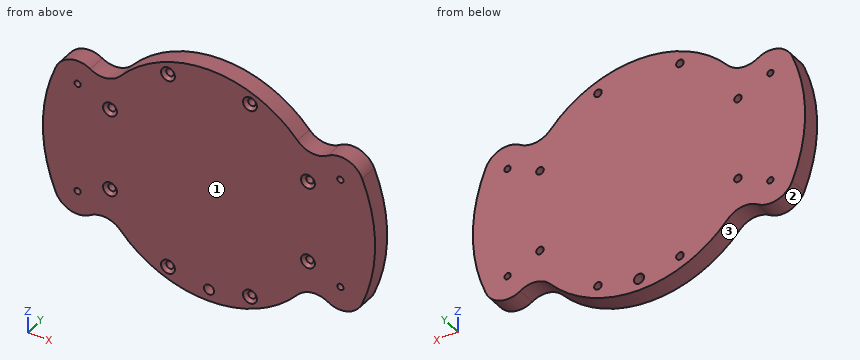
```python
from build123d import *

# Parameters (mm, degrees)
SKETCH1_R                                       = 1
BOSS_EXTRUDE1_DEPTH                             = 6
FILLET1_R                                       = 7.5
SKETCH2_R                                       = 1.6
CUT_EXTRUDE1_DEPTH                              = 66.108380797
CSK_FOR_M2_FLAT_HEAD_MACHINE_SCREW1_D           = 2.4
CSK_FOR_M2_FLAT_HEAD_MACHINE_SCREW1_CSINK_D     = 4.4
CSK_FOR_M2_FLAT_HEAD_MACHINE_SCREW1_CSINK_ANGLE = 90


with BuildPart() as part:
    # Sketch1 → Boss-Extrude1 (new body)
    with BuildSketch(Plane(origin=(0, 0, 0), x_dir=(1, 0, 0), z_dir=(0, 1, 0))):
        with BuildLine():
            Line((31.883633055, 20.164562188), (44.561021943, 28.182280752))
            ThreePointArc((44.561021943, 28.182280752), (52.725, 0), (44.561021943, -28.182280752))
            Line((44.561021943, -28.182280752), (31.883633055, -20.164562188))
            ThreePointArc((31.883633055, -20.164562188), (0, -37.725), (-31.883633055, -20.164562188))
            Line((-31.883633055, -20.164562188), (-44.561021943, -28.182280752))
            ThreePointArc((-44.561021943, -28.182280752), (-52.725, 0), (-44.561021943, 28.182280752))
            Line((-44.561021943, 28.182280752), (-31.883633055, 20.164562188))
            ThreePointArc((-31.883633055, 20.164562188), (0, 37.725), (31.883633055, 20.164562188))
        make_face()
        with Locations(Location((-13.0112367, 31.411904105, 0), (0, 0, 270))):
            Circle(SKETCH1_R, mode=Mode.SUBTRACT)
        with Locations(Location((13.0112367, 31.411904105, 0), (0, 0, 270))):
            Circle(SKETCH1_R, mode=Mode.SUBTRACT)
        with Locations(Location((31.411904105, 13.0112367, 0), (0, 0, 270))):
            Circle(SKETCH1_R, mode=Mode.SUBTRACT)
        with Locations(Location((31.411904105, -13.0112367, 0), (0, 0, 270))):
            Circle(SKETCH1_R, mode=Mode.SUBTRACT)
        with Locations(Location((13.0112367, -31.411904105, 0), (0, 0, 270))):
            Circle(SKETCH1_R, mode=Mode.SUBTRACT)
        with Locations(Location((-13.0112367, -31.411904105, 0), (0, 0, 270))):
            Circle(SKETCH1_R, mode=Mode.SUBTRACT)
        with Locations(Location((-31.411904105, -13.0112367, 0), (0, 0, 270))):
            Circle(SKETCH1_R, mode=Mode.SUBTRACT)
        with Locations(Location((-31.411904105, 13.0112367, 0), (0, 0, 270))):
            Circle(SKETCH1_R, mode=Mode.SUBTRACT)
        with Locations(Location((41.701925915, 17.5, 0), (0, 0, 270))):
            Circle(SKETCH1_R, mode=Mode.SUBTRACT)
        with Locations(Location((41.701925915, -17.5, 0), (0, 0, 270))):
            Circle(SKETCH1_R, mode=Mode.SUBTRACT)
        with Locations(Location((-41.701925915, 17.5, 0), (0, 0, 90))):
            Circle(SKETCH1_R, mode=Mode.SUBTRACT)
        with Locations(Location((-41.701925915, -17.5, 0), (0, 0, 90))):
            Circle(SKETCH1_R, mode=Mode.SUBTRACT)
    extrude(amount=BOSS_EXTRUDE1_DEPTH)

    # Fillet1
    fillet1_edges = [part.edges().sort_by_distance(p)[0] for p in [
        (44.561021943, 3, 28.182280752),
        (31.883633055, 3, 20.164562188),
        (-44.561021943, 3, 28.182280752),
        (-31.883633055, 3, 20.164562188),
        (44.561021943, 3, -28.182280752),
        (31.883633055, 3, -20.164562188),
        (-44.561021943, 3, -28.182280752),
        (-31.883633055, 3, -20.164562188),
    ]]
    fillet(fillet1_edges, radius=FILLET1_R - 0.0001)  # a hair under: the kernel refuses the full size

    # Sketch2 → Cut-Extrude1 (cut, through all)
    with BuildSketch(Plane(origin=(0, 6, 0), x_dir=(1, 0, 0), z_dir=(0, 1, 0))):
        with Locations(Location((0, 34, 0), (0, 0, 270))):
            Circle(SKETCH2_R)
    extrude(amount=-CUT_EXTRUDE1_DEPTH, mode=Mode.SUBTRACT)

    # CSK for M2 Flat Head Machine Screw1 (through all)
    with Locations(Plane(origin=(0, 0, 0), x_dir=(-1, 0, 0), z_dir=(0, -1, 0))):
        with Locations((13.0112367, -31.411904105), (-13.0112367, -31.411904105), (-31.411904105, -13.0112367), (-31.411904105, 13.0112367), (-13.0112367, 31.411904105), (13.0112367, 31.411904105), (31.411904105, 13.0112367), (31.411904105, -13.0112367)):
            CounterSinkHole(CSK_FOR_M2_FLAT_HEAD_MACHINE_SCREW1_D / 2, CSK_FOR_M2_FLAT_HEAD_MACHINE_SCREW1_CSINK_D / 2, counter_sink_angle=CSK_FOR_M2_FLAT_HEAD_MACHINE_SCREW1_CSINK_ANGLE)


solid = part.part
```
The listing builds one solid part. Answer for the finished solid, in the listing's coordinates (mm). Face numbers are marked on the shaded views. Give positions to 0.01 mm unless a question says otherwise; leave off trailing zeros. Write each loop counter-clockwise with the first axis right and the second up, starting at its lowest first coordinate (ties: lowest second). Pieces come first, ordered by that corner, then holes. Notation, with made-up numbers: (3, 68.5) -> (49, 68.5) arc R18 ccw to (49, 91.5) -> close; hole circle Ø7 at (49, 53.25). An arc over 180 degrees is marked (long way). Use one line per item in the form item = value.
1) Each of these flat-tipped pins is pushed along its axis until it touches: P1, Ø4, axis at x = 13.01, z = 31.41, coming from the -Y side; P2, Ø3, axis at y = 2, z = 3, coming from the -X side; P3, Ø1, axis at x = 27.5, y = 4.5, coming from the -Z side. Where does it stop, or does it pass through?
Result:
P1 = 0.2
P2 = -52.7
P3 = -26.35
2) Section A-A on x = 0 is taken. Write down the section's boundary in (y, z) (3 decimals), plus the area to 4 significant figures.
Result:
outline = (0, -37.725) -> (6, -37.725) -> (6, -35.6) -> (0, -35.6) -> close; (0, -32.4) -> (6, -32.4) -> (6, 37.725) -> (0, 37.725) -> close
area = 433.5 mm²
3) For a pull along X with two mould halves and no side action, classify the marked faces 1, 2 and 3 as +X half, -X half, draft (parallel to the pull), parting line (faces both ways), or undercut.
Result:
face_1 = draft
face_2 = undercut
face_3 = parting line
4) Straight lines are drawn through the part: probe 1 along X at (y, z) = (2.8, 17.5); probe 2 along X at (y, z) = (3.85, -13); probe 3 along Z at (x, y) = (-13.5, 2.75). For each, find the intervals that lie inside material, in ascending order.
Result:
probe_1 = -49.74 to -42.7, -40.7 to 40.7, 42.7 to 49.74
probe_2 = -51.1 to -32.61, -30.21 to 30.21, 32.61 to 51.1
probe_3 = -35.23 to -32.51, -30.32 to 30.32, 32.51 to 35.23
5) Section C-C on z = -28 is taken. Write down the section's boundary in (x, y), plus the area to 3 significant figures.
Result:
outline = (-25.28, 0) -> (25.28, 0) -> (25.28, 6) -> (-25.28, 6) -> close
area = 303 mm²
6) Section B-B on y = 4.2 is taken. Count the separate pieces of the cut face and the enclosed holes in it, plus the area to 3 significant figures.
Result:
separate_pieces = 1
enclosed_holes = 13
area = 5,920 mm²
7) Section D-D on x = -36 is taken. Write down the section's boundary in (y, z), plus the area to 3 significant figures.
Result:
outline = (0, -23.04) -> (6, -23.04) -> (6, 23.04) -> (0, 23.04) -> close
area = 277 mm²
